```python
from build123d import *

# Parameters (mm, degrees)
ESBO_O1_R                = 24.5
ESBO_O1_R_2              = 18
ESBO_O1_R_3              = 3.5
RESSALTO_EXTRUS_O1_DEPTH = 9
ESBO_O2_R                = 18
CORTE_EXTRUS_O1_DEPTH    = 2
CORTE_EXTRUS_O1_TAPER    = 45


with BuildPart() as part:
    # Esboço1 → Ressalto-extrusão1 (new body)
    # profile 1 of 2: a face of its own
    with BuildSketch(Plane.XY):
        with Locations((-21.997899875, 9.443861076)):
            Circle(ESBO_O1_R)
        with Locations((-21.997899875, 9.443861076)):
            Circle(ESBO_O1_R_2, mode=Mode.SUBTRACT)
    # profile 2 of 2: a face of its own
    with BuildSketch(Plane.XY):
        with Locations((-21.997899875, 9.443861076)):
            Circle(ESBO_O1_R_2)
        with Locations((-33.997899875, 9.443861076)):
            Circle(ESBO_O1_R_3, mode=Mode.SUBTRACT)
        with Locations((-21.997899875, 21.443861076)):
            Circle(ESBO_O1_R_3, mode=Mode.SUBTRACT)
        with Locations((-9.997899875, 9.443861076)):
            Circle(ESBO_O1_R_3, mode=Mode.SUBTRACT)
        with Locations((-21.997899875, -2.556138924)):
            Circle(ESBO_O1_R_3, mode=Mode.SUBTRACT)
        with Locations((-21.997899875, 9.443861076)):
            Circle(ESBO_O1_R_3, mode=Mode.SUBTRACT)
    extrude(amount=RESSALTO_EXTRUS_O1_DEPTH)

    # Esboço2 → Corte-extrusão1 (cut)
    with BuildSketch(Plane.XY):
        with Locations((-21.997899875, 9.443861076)):
            Circle(ESBO_O2_R)
    extrude(amount=CORTE_EXTRUS_O1_DEPTH, taper=CORTE_EXTRUS_O1_TAPER, mode=Mode.SUBTRACT)


solid = part.part
```
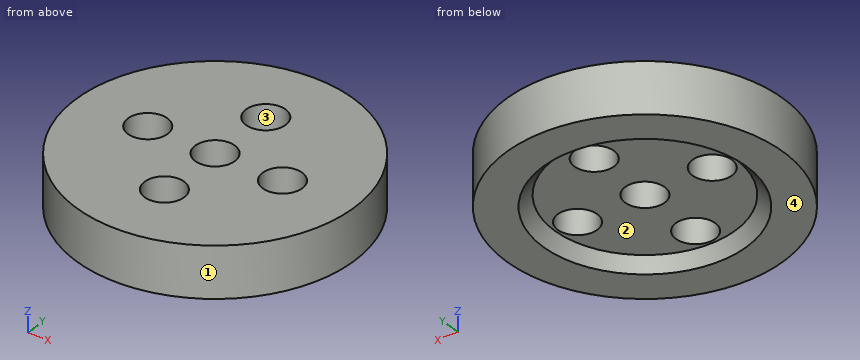
The model under review builds one solid part; all positions refer to its coordinate system, in mm. Face numbers are marked on the shaded views. Round coordinates to 2 decimals unless told otherwise and drop trailing zeros. Loops run counter-clockwise (first coordinate to the right, second up) from the corner with the lowest first, then second, coordinate; pieces in that order, holes last.
1) Consider section B-B on x = -24.5. Give the number of separate pieces and of enclosed holes in the cut face, then the cut area to 3 significant figures.
Values follow:
separate pieces: 4
enclosed holes: 0
area: 269 mm2
2) Consider section C-C on y = -12. State the section outline as (x, z) points.
Values follow:
outline: (-33.85, 0) - (-10.15, 0) - (-10.15, 9) - (-33.85, 9) - close
3) Wall thickness on line 1 along X through (y, z) = (9.5, 5); line 2 along X through (y, z) = (8, 6.5); line 3 along Z through (x, y) = (-18, 20.5): over which ranges is each line inside the solid? List them lowest first.
Values follow:
line 1: x = -46.5 to -37.5, -30.5 to -25.5, -18.5 to -13.5, -6.5 to 2.5
line 2: x = -46.46 to -37.19, -30.81 to -25.19, -18.81 to -13.19, -6.81 to 2.46
line 3: z = 2 to 9
4) The part is to be moulded in two halves that separate along Y. For the marked faces 1, 2, 3 and 4, say which applies: pulls with the +Y half, pulls with the -Y half, needs draft (parallel to the pull), parting line crosses it, or undercut.
Values follow:
face 1: parting line crosses it
face 2: undercut
face 3: undercut
face 4: needs draft
5) Clearance check with flat-ended pins moving along their axes: P1, Ø4, axis at y = -5.5, z = 3, coming from the +X side; P2, Ø16, axis at x = -20.5, y = 8, coming from the -Z side; P3, Ø5, axis at y = 26.5, z = 3.5, coming from the +X side. State where each tip first meets the part, or that it passes through.
Values follow:
P1: stops at x = -1.2
P2: stops at z = 2
P3: stops at x = -2.29
6) Consider section A-A on z = 7. State the section outline as (x, y) points, then the cut area to 3 significant figures.
Values follow:
outline: circle Ø49 at (-22, 9.44); hole circle Ø7 at (-34, 9.44); hole circle Ø7 at (-22, -2.56); hole circle Ø7 at (-22, 9.44); hole circle Ø7 at (-22, 21.44); hole circle Ø7 at (-10, 9.44)
area: 1,690 mm2
7) Consider section D-D on z = 1.25. State the section outline as (x, y) points, then the cut area to 3 significant figures.
Values follow:
outline: circle Ø49 at (-22, 9.44); hole circle Ø33.5 at (-22, 9.44)
area: 1,000 mm2
